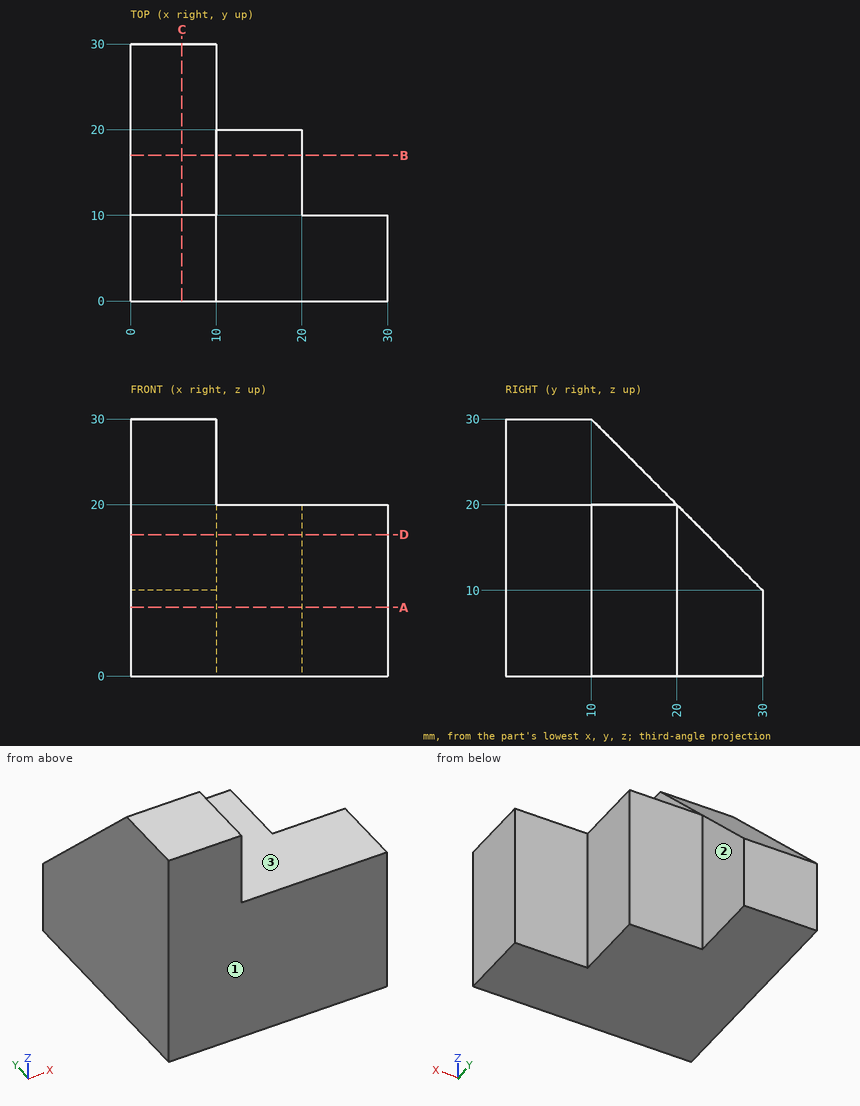
Could you check a few things on this drawing? It's one solid part, dimensions in mm from its lowest x, y, z. A direction names the side the tool comes from. Round coordinates to 2 decimals unless told otherwise and drop trailing zeros. Write each loop counter-clockwise with the first axis right and the second up, starting at its lowest first coordinate (ties: lowest second). Pieces come first, ordered by that corner, then holes. Notation, with made-up numbers: (-22.5, 50.25) -> (11.5, 50.25) arc R33 cw to (11.5, 86.25) -> close; hole circle Ø11 at (11, -35). An arc over 180 degrees is marked (long way). One line per item, written item: value.
1) Suppose I cut it at B-B on y = 17. List the corners of the cut face in (x, z) for me.
Filled sheet:
outline: (0, 0) -> (20, 0) -> (20, 20) -> (10, 20) -> (10, 23) -> (0, 23) -> close
2) Suppose I cut it at C-C on x = 6. List the corners of the cut face in (y, z) for me.
Filled sheet:
outline: (0, 0) -> (30, 0) -> (30, 10) -> (10, 30) -> (0, 30) -> close
3) If I drill on line 1 (X direction, y = 14, z = 17.25), over which ranges is the centre line in solid material (lowest first)? Write a range as [from, to].
Filled sheet:
line 1: x = [0, 20]
4) Suppose I cut it at A-A on z = 8. List the corners of the cut face in (x, y) for me.
Filled sheet:
outline: (0, 0) -> (30, 0) -> (30, 10) -> (20, 10) -> (20, 20) -> (10, 20) -> (10, 30) -> (0, 30) -> close
5) I'm going to push flat-ended pins straight in: pin 1 Ø11 at (x, z) = (27.5, 8) entering from +Y; pin 2 Ø3 at (y, z) = (14.5, 20) entering from +X; pin 3 Ø1 at (x, z) = (17.5, 10) entering from -Y; pin 4 Ø3 at (y, z) = (10, 26.5) entering from +X. Where does each tip first touch, or does it pass through?
Filled sheet:
pin 1: stops at y = 10
pin 2: stops at x = 20
pin 3: stops at y = 0
pin 4: stops at x = 10
6) Suppose I cut it at D-D on z = 16.5. List the corners of the cut face in (x, y) for me, plus the area to 3 significant figures.
Filled sheet:
outline: (0, 0) -> (30, 0) -> (30, 10) -> (20, 10) -> (20, 20) -> (10, 20) -> (10, 23.5) -> (0, 23.5) -> close
area: 535 mm2
7) For the marked faces 1, 2 and 3, which set-ups out of +Z, -Z, +X, -X, +Y, -Y let a thin tool reach every point of the face, with its end or its side?
Filled sheet:
face 1: +Z, -Z, +X, -X, -Y
face 2: +Z, -Z, +X, +Y
face 3: +Z, +X, +Y, -Y
